For this review, take the finished solid that the model builds, in its own axes (mm). Round coordinates to 2 decimals unless told otherwise and drop trailing zeros. Order: outer loops, then holes, each group sorted by start corner. A loop starts at its lowest first (then second) coordinate and runs counter-clockwise, first axis right, second up. Notation, with made-up numbers: M 70,6.5 L 98,6.5 A19 cw 98,32.5 Z; hole C 57,-28.75 d9. An arc over 180 degrees is marked long. Write item = value, one per line. Start each with the question number.
from build123d import *

# Parameters (mm, degrees)
SKETCH3_W           = 156.21
SKETCH3_H           = 55.88
BOSS_EXTRUDE2_DEPTH = 2.032
SKETCH4_W           = 151.888767811
SKETCH4_H           = 63.5
BOSS_EXTRUDE3_DEPTH = 3.048
SKETCH5_W           = 13.94179759
SKETCH5_H           = 16.111517863
CUT_EXTRUDE1_DEPTH  = 6.08


with BuildPart() as part:
    # Sketch3 → Boss-Extrude2 (new body)
    with BuildSketch(Plane.XY):
        with Locations((75.809845761, 22.583067422)):
            Rectangle(SKETCH3_W, SKETCH3_H)
    extrude(amount=BOSS_EXTRUDE2_DEPTH)

    # Sketch4 → Boss-Extrude3 (add)
    with BuildSketch(Plane.XY.offset(2.032)):
        with Locations((77.970461856, 22.583067422)):
            Rectangle(SKETCH4_W, SKETCH4_H)
    extrude(amount=BOSS_EXTRUDE3_DEPTH)

    # Sketch5 → Cut-Extrude1 (cut, through all)
    with BuildSketch(Plane.XY.offset(5.08)):
        with Locations((146.943946966, 23.09296993)):
            Rectangle(SKETCH5_W, SKETCH5_H)
    extrude(amount=-CUT_EXTRUDE1_DEPTH, mode=Mode.SUBTRACT)


solid = part.part
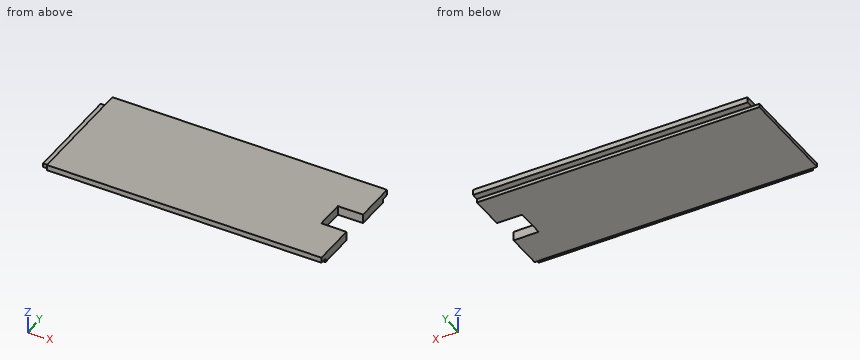
(1) Insertion check: pin 1 (3 mm diameter, centred on x = 61, y = 51.5, fed in from -Z); pin 2 (1.6 mm diameter, centred on x = 106, z = 1, fed in from +Y); pin 3 (0.9 mm diameter, centred on y = 17.5, z = 3.5, fed in from -X); pin 4 (1.5 mm diameter, centred on y = 19.5, z = 3.5, fed in from +X). Each pin has a flat end and moves straight along its axis. Give the tip position at first contact, or say it passes through.
(2) For line 1 along X through (y, z) = (-6, 2.35); line 2 along Y through (x, z) = (97, 1.75); line 3 along Z through (x, y) = (46.5, -6.5), list the stretches that pass through material, from the lowest coordinate up.
(3) We need section D-D, the plane y = 16.5. Write out the cut boundary in (x, z).
(4) We need section B-B, the plane y = 48. Write out the cut boundary in (x, z).
(5) We need section A-A, the plane z = 3.75. Write out the cut boundary in (x, y).
(6) We need section C-C, the plane x = 95. Write out the cut boundary in (y, z), then the cut area to 3 significant figures.
Values:
q1.pin_1 = 0
q1.pin_2 = 50.52
q1.pin_3 = 2.03
q1.pin_4 = 139.97
q2.line_1 = 2.03 to 153.91
q2.line_2 = -5.36 to 50.52
q2.line_3 = 2.03 to 5.08
q3.outline = M -2.3,0 L 139.97,0 L 139.97,5.08 L 2.03,5.08 L 2.03,2.03 L -2.3,2.03 Z
q4.outline = M -2.3,0 L 153.91,0 L 153.91,5.08 L 2.03,5.08 L 2.03,2.03 L -2.3,2.03 Z
q5.outline = M 2.03,-9.17 L 153.91,-9.17 L 153.91,15.04 L 139.97,15.04 L 139.97,31.15 L 153.91,31.15 L 153.91,54.33 L 2.03,54.33 Z
q6.outline = M -9.17,2.03 L -5.36,2.03 L -5.36,0 L 50.52,0 L 50.52,2.03 L 54.33,2.03 L 54.33,5.08 L -9.17,5.08 Z
q6.area = 307 mm²
